```python
from build123d import *

# Parameters (mm, degrees)
SKETCH_1_W          = 30
SKETCH_1_H          = 50
EXTRUDE_1_DEPTH     = 3
SKETCH_2_R          = 7
SKETCH_2_R_2        = 2.1
CUT_EXTRUDE_1_DEPTH = 59.386642308


with BuildPart() as part:
    # 草图1 → 凸台-拉伸1 (new body)
    with BuildSketch(Plane.XY):
        with Locations((15, -25)):
            Rectangle(SKETCH_1_W, SKETCH_1_H)
    extrude(amount=EXTRUDE_1_DEPTH)

    # 草图2 → 切除-拉伸1 (cut, through all)
    with BuildSketch(Plane.XY.offset(3)):
        with Locations((10, -25)):
            Circle(SKETCH_2_R)
        with Locations((25, -10)):
            Circle(SKETCH_2_R_2)
        with Locations(Location((25, -40, 0), (0, 0, 180))):
            Circle(SKETCH_2_R_2)
    extrude(amount=-CUT_EXTRUDE_1_DEPTH, mode=Mode.SUBTRACT)


solid = part.part
```
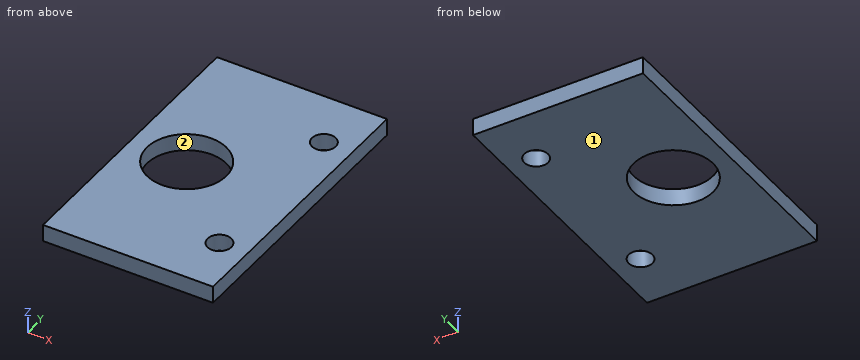
Can you work these out from the model? Positions are in its coordinate system, mm. Face numbers are marked on the shaded views. Round coordinates to 2 decimals unless told otherwise and drop trailing zeros. Loops run counter-clockwise (first coordinate to the right, second up) from the corner with the lowest first, then second, coordinate; pieces in that order, holes last. Notation, with made-up numbers: (68.5, -19) -> (110.5, -19) arc R23 ccw to (110.5, 16) -> close; hole circle Ø10 at (20.25, 71.5). An arc over 180 degrees is marked (long way). Answer in a Markdown table with one row per item.
Item 1: If I drill on probe 1 along X at (y, z) = (-40, 1); probe 2 along Y at (x, z) = (25, 1.65); probe 3 along Y at (x, z) = (9.75, 1.65), over which ranges is the centre line in solid material (lowest first)?
Answer block:
| item | result |
|---|---|
| probe 1 | 0 to 22.9, 27.1 to 30 |
| probe 2 | -50 to -42.1, -37.9 to -12.1, -7.9 to 0 |
| probe 3 | -50 to -32, -18 to 0 |
Item 2: Suppose I cut it at D-D, the plane y = -40. List the corners of the cut face in (x, z) for me, plus the area to 3 significant figures.
Answer block:
| item | result |
|---|---|
| outline | (0, 0) -> (22.9, 0) -> (22.9, 3) -> (0, 3) -> close; (27.1, 0) -> (30, 0) -> (30, 3) -> (27.1, 3) -> close |
| area | 77.4 mm² |
Item 3: Suppose I cut it at B-B, the plane y = -25. List the corners of the cut face in (x, z) for me, plus the area to 3 significant figures.
Answer block:
| item | result |
|---|---|
| outline | (0, 0) -> (3, 0) -> (3, 3) -> (0, 3) -> close; (17, 0) -> (30, 0) -> (30, 3) -> (17, 3) -> close |
| area | 48.0 mm² |
Item 4: We'd pull the mould along X, two halves only. Please class the marked faces 1 and 2: released by +X, released by -X, zero draft, split by the parting line, or undercut.
Answer block:
| item | result |
|---|---|
| face 1 | zero draft |
| face 2 | undercut |
Item 5: Suppose I cut it at C-C, the plane z = 1.4. List the corners of the cut face in (x, y) for me, plus the area to 3 significant figures.
Answer block:
| item | result |
|---|---|
| outline | (0, -50) -> (30, -50) -> (30, 0) -> (0, 0) -> close; hole circle Ø14 at (10, -25); hole circle Ø4.2 at (25, -40); hole circle Ø4.2 at (25, -10) |
| area | 1,320 mm² |
Item 6: Will these pins go through, and if not, where does the flat tip stop? P1, Ø11, axis at x = 10, y = -25, coming from the -Z side; P2, Ø5, axis at x = 7, y = -45, coming from the -Z side.
Answer block:
| item | result |
|---|---|
| P1 | through |
| P2 | z = 0 |
Item 7: Suppose I cut it at A-A, the plane x = 25. List the corners of the cut face in (y, z) for me.
Answer block:
| item | result |
|---|---|
| outline | (-50, 0) -> (-42.1, 0) -> (-42.1, 3) -> (-50, 3) -> close; (-37.9, 0) -> (-12.1, 0) -> (-12.1, 3) -> (-37.9, 3) -> close; (-7.9, 0) -> (0, 0) -> (0, 3) -> (-7.9, 3) -> close |
